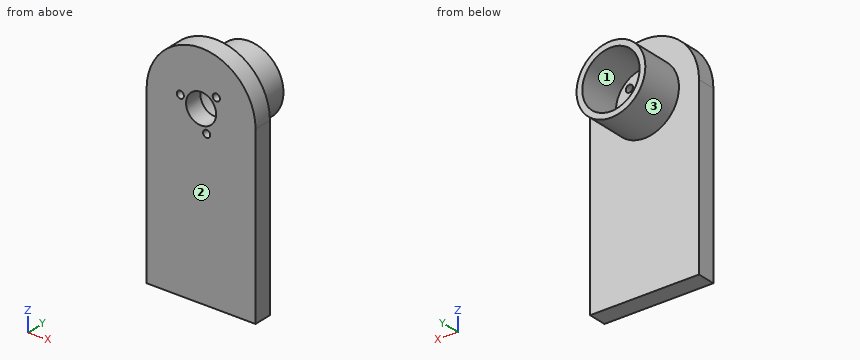
```python
from build123d import *

# Parameters (mm, degrees)
F1_DEPTH        = 6.4
F2_R            = 1.25
F3_DEPTH        = 6.401
F3_COPIES_COUNT = 3
F4_R            = 5.25
F5_DEPTH        = 6.401
F6_R            = 12
F6_R_2          = 10
F7_DEPTH        = 15


# Not quite as in the source:
# - a pattern or mirror of a feature is missing from the dataset's text; its kind, count and spacing are read off the source's solid


with BuildPart() as f1:
    # F0 (on Front) → F1 (new body)
    with BuildSketch(Plane.XZ):
        with BuildLine():
            Line((-19, 0), (-19, -61))
            Line((-19, -61), (19, -61))
            Line((19, -61), (19, 0))
            ThreePointArc((19, 0), (0, 19), (-19, 0))
        make_face()
    extrude(amount=F1_DEPTH)

    # F2 (on Front) → F3 (cut, through all)
    with BuildSketch(Plane.XZ):
        with Locations((5.3033008589, 5.3033008589)):
            Circle(F2_R)
    f3 = extrude(amount=F3_DEPTH, mode=Mode.SUBTRACT)

    # F3_copies: F3 ×3 about axis
    f3_copies_axis = Axis((0, 0, 0), (0, 1, 0))
    for i in range(1, F3_COPIES_COUNT):
        add(f3.rotate(f3_copies_axis, i * 360 / F3_COPIES_COUNT), mode=Mode.SUBTRACT)

    # F4 (on Front) → F5 (cut, through all)
    with BuildSketch(Plane.XZ):
        Circle(F4_R)
    extrude(amount=F5_DEPTH, mode=Mode.SUBTRACT)

    # F6 (on face) → F7 (join)
    with BuildSketch(Plane(origin=(0, 0, 0), x_dir=(-1, 0, 0), z_dir=(0, 1, 0))):
        Circle(F6_R)
        Circle(F6_R_2, mode=Mode.SUBTRACT)
    extrude(amount=F7_DEPTH)


solid = f1.part
```
Part model, mm, in its own coordinate system. Face numbers are marked on the shaded views. Round coordinates to 2 decimals unless told otherwise and drop trailing zeros. Write each loop counter-clockwise with the first axis right and the second up, starting at its lowest first coordinate (ties: lowest second). Pieces come first, ordered by that corner, then holes. Notation, with made-up numbers: (12.5, 33) -> (35.5, 33) arc R14 ccw to (35.5, 48) -> close; hole circle Ø5 at (-38.5, 3.5). An arc over 180 degrees is marked (long way). Return JSON: item names as keys, results as strings. Group by question number.
Q1. Saw through at D-D on y = 7.5. Write the cut outline in (x, z).
Q2. Saw through at B-B on y = -4.75. Write the cut outline in (x, z), plus the area to 3 significant figures.
Q3. Mould opens along Z. For the marked faces 1, 2 and 3 say: pulls with the +Z half, pulls with the -Z half, needs draft (parallel to the pull), parting line crosses it, or undercut.
Q4. Saw through at C-C on x = 9. Write the cut outline in (y, z), plus the area to 3 significant figures.
Q5. Probe L1, parallel to Z at x = 0, y = 4.5; L2, parallel to Y at x = 7.5, z = -1.5; L3, parallel to Z at x = 2.5, y = 3.25. List the from-to ranges inside material, lowest first. Write a range as [from, to].
Q6. Saw through at A-A on z = -7. Write the cut outline in (x, y), plus the area to 3 significant figures.
Q7. Pin check, flat tips, straight feed: pin 1 (2 mm diameter, centred on y = -1.5, z = 3.5, fed in from +X); pin 2 (4 mm diameter, centred on x = 1.94, z = -7.24, fed in from +Y); pin 3 (3 mm diameter, centred on x = -11, y = 2, fed in from +Z). Stop position of each tip, or through.
Answer:
{
 "1": {"outline": "circle Ø24 at (0, 0); hole circle Ø20 at (0, 0)"},
 "2": {"outline": "(-19, -61) -> (19, -61) -> (19, 0) arc R19 ccw to (-19, 0) -> close; hole circle Ø2.5 at (-7.24, 1.94); hole circle Ø10.5 at (0, 0); hole circle Ø2.5 at (1.94, -7.24); hole circle Ø2.5 at (5.3, 5.3)", "area": "2,780 mm2"},
 "3": {"face 1": "undercut", "face 2": "needs draft", "face 3": "parting line crosses it"},
 "4": {"outline": "(-6.4, -61) -> (0, -61) -> (0, -7.94) -> (15, -7.94) -> (15, -4.36) -> (0, -4.36) -> (0, 4.36) -> (15, 4.36) -> (15, 7.94) -> (0, 7.94) -> (0, 16.73) -> (-6.4, 16.73) -> close", "area": "605 mm2"},
 "5": {"L1": "[-12, -10], [10, 12]", "L2": "[-6.4, 0]", "L3": "[-11.74, -9.68], [9.68, 11.74]"},
 "6": {"outline": "(-19, -6.4) -> (0.72, -6.4) -> (0.72, 0) -> (-7.14, 0) -> (-7.14, 15) -> (-9.75, 15) -> (-9.75, 0) -> (-19, 0) -> close; (3.17, -6.4) -> (19, -6.4) -> (19, 0) -> (9.75, 0) -> (9.75, 15) -> (7.14, 15) -> (7.14, 0) -> (3.17, 0) -> close", "area": "306 mm2"},
 "7": {"pin 1": "x = 18.83", "pin 2": "y = 0", "pin 3": "z = 7.33"}
}
